Read the model definition and answer for the solid it produces. Units are mm, in the model's axes. A direction names the side the tool comes from. Give positions to 0.01 mm unless a question says otherwise; leave off trailing zeros. Write each loop counter-clockwise with the first axis right and the second up, starting at its lowest first coordinate (ties: lowest second). Pieces come first, ordered by that corner, then holes. Notation, with made-up numbers: (-8.75, 80) -> (20.25, 80) arc R8 cw to (20.25, 85) -> close; hole circle Ø1 at (-30.75, 13). An arc over 180 degrees is marked (long way). Put each result on its own line as item: value. Start each with the question number.
from build123d import *

# Parameters (mm, degrees)
F1_DEPTH = 60
F0_W     = 90
F0_H     = 70
F2_DEPTH = 10
F3_DEPTH = 90
F5_START = 45
F5_DEPTH = 5
F6_START = -45
F6_DEPTH = 5


with BuildPart() as f1:
    # F0 (on Top) → F1 (new body)
    with BuildSketch(Plane.XY):
        Polygon((45, -35), (50, -35), (50, 40), (-50, 40), (-50, -35), (-45, -35), (-45, 35), (45, 35), align=None)
    extrude(amount=F1_DEPTH)

    # F0 (on Top) → F2 (join)
    with BuildSketch(Plane.XY):
        Rectangle(F0_W, F0_H)
    extrude(amount=F2_DEPTH)

    # F0 (on Top) → F3 (join)
    with BuildSketch(Plane.XY):
        Polygon((-50, -40), (50, -40), (50, -35), (45, -35), (-45, -35), (-50, -35), align=None)
    extrude(amount=F3_DEPTH)

    # F4 (on Right) → F5 (join)
    with BuildSketch(Plane.YZ.offset(F5_START)):
        Polygon((-35.0263789296, 89.9869129062), (-35.307901961, 59.999383986), (39.9987436831, 59.999383986), align=None)
    extrude(amount=F5_DEPTH)

    # F4 (on Right) → F6 (join)
    with BuildSketch(Plane.YZ.offset(F6_START)):
        Polygon((-35.0263789296, 89.9869129062), (-35.307901961, 59.999383986), (39.9987436831, 59.999383986), align=None)
    extrude(amount=-F6_DEPTH)


solid = f1.part
1) For a pull along Y with two mould halves and no side action, classify faces 4 (the face through (1, -35, 49)), 5 (the face through (-1, 1, 0)), 6 (the face through (-47.46, 3.02, 74.78)) as pulls with the +Y half, pulls with the -Y half, needs draft (parallel to the pull), parting line crosses it, or undercut.
2) Straight lines are drawn through the part: line 1 (X direction, y = -19, z = 72.5); line 2 (Y direction, x = -24.5, z = 42); line 3 (Z direction, x = 30.5, y = -13). For each, find the intervals that lie inside material, in ascending order. Write a range as [from, to].
3) A cutting plane is placed at B-B on x = 31. Give the vertices of the cut face in (y, z).
4) A cutting plane is placed at C-C on y = -32. Give the vertices of the cut face in (x, z).
5) Each of these flat-tipped pins is pushed along its axis until it touches: pin 1 Ø1.5 at (x, y) = (2, 23) entering from +Z; pin 2 Ø2.5 at (x, y) = (-17.5, 38) entering from +Z. Where does it stop, or does it pass through?
6) For faces 1 (the face through (47.46, 3.02, 74.78)), 2 (the face through (-1, 38, 60)), 3 (the face through (-1, 35, 35)), determine the directions among +Z, -Z, +X, -X, +Y, -Y from which every point of the face is accessible in a straight line to the end or side of a thin tool.
7) A cutting plane is placed at A-A on z = 56. Give the vertices of the cut face in (x, y), and give its area (3 significant figures).
Results found:
1. face 4: undercut
1. face 5: needs draft
1. face 6: pulls with the +Y half
2. line 1: x = [-50, -45], [45, 50]
2. line 2: y = [-40, -35], [35, 40]
2. line 3: z = [0, 10]
3. outline: (-40, 0) -> (40, 0) -> (40, 60) -> (35, 60) -> (35, 10) -> (-35, 10) -> (-35, 90) -> (-40, 90) -> close
4. outline: (-50, 0) -> (50, 0) -> (50, 88.78) -> (45, 88.78) -> (45, 10) -> (-45, 10) -> (-45, 88.78) -> (-50, 88.78) -> close
5. pin 1: stops at z = 10
5. pin 2: stops at z = 60
6. face 1: +Z, +X, -X, +Y
6. face 2: +Z, +Y
6. face 3: +Z
7. outline: (-50, -40) -> (50, -40) -> (50, 40) -> (-50, 40) -> close; hole (-45, -35) -> (45, -35) -> (45, 35) -> (-45, 35) -> close
7. area: 1,700 mm²
